Autodesk Inventor part; units mm, degrees
ref_plane "YZ Plane" through (0, 0, 0) normal (1, 0, 0) x (0, 1, 0)
ref_plane "XZ Plane" through (0, 0, 0) normal (0, 1, 0) x (-1, 0, 0)
ref_plane "XY Plane" through (0, 0, 0) normal (0, 0, 1) x (1, 0, 0)
sketch "Sketch1" plane through (0, 0, 0) normal (0, 1, 0) x (-1, 0, 0)
  line L0 (30, -20) -> (-30, -20)
  line L1 (-30, -20) -> (-30, 20)
  line L2 (-30, 20) -> (30, 20)
  line L3 (30, 20) -> (30, -20)
  line L4 (30, -20) -> (-30, 20) construction
  line L5 (-30, -20) -> (30, 20) construction
  point P0 (0, 0)
  dimension "d0" = 60
  dimension "d1" = 40
extrude "Extrusion1" add sketch "Sketch1" along normal blind 5.5
sketch "Sketch2" plane through (0, 5.5, 0) normal (0, 1, 0) x (1, 0, 0)
  line L0 (30, -20) -> (30, 20)
  line L1 (30, 0) -> (43.5, 0)
  line L2 (43.5, 0) -> (43.5, 10)
  line L3 (43.5, 10) -> (30, 10)
  line L4 (30, 10) -> (30, 0)
  line L5 (-43.1, 0) -> (48.6, 0)
  line L6 (43.5, 0) -> (43.5, -10)
  line L7 (43.5, -10) -> (30, -10)
  line L8 (30, -10) -> (30, 0)
  point P0 (0, 0)
  dimension "d4" = 13.5
  dimension "d5" = 10
extrude "Extrusion2" add sketch "Sketch2" against normal blind 5.5
sketch "Sketch3" plane through (0, 5.5, 0) normal (0, 1, 0) x (1, 0, 0)
  line L0 (43.5, 10) -> (30, 10)
  line L1 (30, 10) -> (30, 20)
  line L2 (35.5, 10) -> (38.5, 10)
  line L3 (38.5, 10) -> (38.5, 0)
  line L4 (38.5, 0) -> (35.5, 0)
  line L5 (35.5, 0) -> (35.5, 10)
  point P0 (0, 0)
  dimension "d8" = 5.5
  dimension "d9" = 3
  dimension "d10" = 10
extrude "Extrusion3" cut sketch "Sketch3" against normal through all
sketch "Sketch4" plane through (0, 5.5, 0) normal (0, 1, 0) x (1, 0, 0)
  line L0 (35.5, 0) -> (35.5, 10)
  line L1 (35.5, 10) -> (30, 10)
  line L2 (30, 10) -> (30, 20)
  line L3 (30, 20) -> (-30, 20)
  line L4 (-30, 20) -> (-30, -20)
  line L5 (-30, -20) -> (30, -20)
  line L6 (30, -20) -> (30, -10)
  line L7 (30, -10) -> (43.5, -10)
  line L8 (43.5, -10) -> (43.5, 10)
  line L9 (43.5, 10) -> (38.5, 10)
  line L10 (38.5, 10) -> (38.5, 0)
  line L11 (38.5, 0) -> (35.5, 0)
  point P0 (0, 0)
sketch "Sketch5" plane through (0, 5.5, 0) normal (0, 1, 0) x (1, 0, 0)
  line L0 (-30, 20) -> (-30, -20)
  line L1 (-44.7, 0) -> (58.2, 0)
  line L2 (0, 28) -> (0, -28)
  line L3 (-30, 0) -> (-41, 0)
  line L4 (-41, 0) -> (-41, 10)
  line L5 (-41, 10) -> (-30, 10)
  line L6 (-30, 10) -> (-30, 0)
  line L7 (-30, 0) -> (-41, 0)
  line L8 (-41, 0) -> (-41, -20)
  line L9 (-41, -20) -> (-30, -20)
  line L10 (-30, -20) -> (-30, 0)
  point P0 (0, 0)
  dimension "d14" = 11
  dimension "d15" = 10
extrude "Extrusion4" add sketch "Sketch5" against normal blind 5.5
sketch "Sketch6" plane through (0, 5.5, 0) normal (0, 1, 0) x (1, 0, 0)
  line L0 (-30, 20) -> (-30, 10)
  line L1 (-30, 10) -> (-41, 10)
  line L2 (-30, 0) -> (-35.5, 0)
  line L3 (-35.5, 0) -> (-35.5, 10)
  line L4 (-35.5, 10) -> (-30, 10)
  line L5 (-30, 10) -> (-30, 0)
  line L6 (-57.9, 0) -> (60.4, 0)
  line L7 (0, 28) -> (0, -28)
  point P0 (0, 0)
  dimension "d20" = 0
  dimension "d21" = 5.5
extrude "Extrusion5" cut sketch "Sketch6" against normal through all
equation "\"d2\" = Wt"
equation "\"d6\" = Wt"
equation "\"d8\" = Wt"
equation "\"d11\" = Wt"
equation "\"d14\" = 2 * Wt"
equation "\"d16\" = Wt"
equation "\"d21\" = Wt"
equation "\"d22\" = Wt"
properties part number "ex_holder_side" material "Wood (Birch)"
Source: CAD feature listing. Evaluate the final solid. Frame: model axes, mm. A direction names the side the tool comes from. Give positions to 0.01 mm unless a question says otherwise; leave off trailing zeros. Write each loop counter-clockwise with the first axis right and the second up, starting at its lowest first coordinate (ties: lowest second). Pieces come first, ordered by that corner, then holes. Notation, with made-up numbers: (71.25, 32) - (128.25, 32) arc R25 ccw to (128.25, 51) - close; hole circle Ø10 at (77, 58). An arc over 180 degrees is marked (long way). One line per item, written item: value. Start each with the question number.
Q1. Draft query along X for faces 4 (the face through (-33, 3, 0)), 5 (the face through (0, 3, -20)), 6 (the face through (30, 3, 15)), 7 (the face through (35.5, 3, -5)). Return one class per face: +X half, -X half, draft (parallel to the pull), parting line (faces both ways), or undercut.
Q2. Section query B-B, the plane x = 32. Return the cut outline in (y, z), then the cut area to 3 significant figures.
Q3. Section query A-A, the plane y = 2.85. Return the cut outline in (x, z), then the cut area to 4 significant figures.
Q4. Material intervals for probe 1 along X at (y, z) = (1.75, -0.5); probe 2 along X at (y, z) = (0.7, 11.5); probe 3 along Z at (x, y) = (-32, 3.8), sorted ascending. Write a range as from..to.
Q5. Set-up query: faces 1 (the face through (37, 3, 10)), 2 (the face through (-30, 3, -10)), 3 (the face through (30, 3, -15)). Return all of +Z, -Z, +X, -X, +Y, -Y with unobstructed straight access to the full face (end or side cutting, diameter ignored); none if empty.
Q6. First-contact query: pin 1 Ø3 at (y, z) = (2, -14.5) entering from -X; pin 2 Ø2 at (x, z) = (2.5, 5.5) entering from -Y; pin 3 Ø1.5 at (x, y) = (37, 3.5) entering from -Z; pin 4 Ø3 at (x, y) = (40, 2.5) entering from +Z. Flat tips, straight axial feed; report the tip coordinate or a pass-through.
Q7. Section query C-C, the plane z = -16. Return the cut outline in (x, y), then the cut area to 3 significant figures.
Answer:
1. face 4: undercut
1. face 5: draft
1. face 6: +X half
1. face 7: undercut
2. outline: (0, -10) - (5.5, -10) - (5.5, 10) - (0, 10) - close
2. area: 110 mm2
3. outline: (-41, -10) - (-35.5, -10) - (-35.5, 0) - (-30, 0) - (-30, -20) - (30, -20) - (30, -10) - (35.5, -10) - (35.5, 0) - (38.5, 0) - (38.5, -10) - (43.5, -10) - (43.5, 10) - (30, 10) - (30, 20) - (-41, 20) - close
3. area: 2,915 mm2
4. probe 1: x = -41..-35.5, -30..35.5, 38.5..43.5
4. probe 2: x = -41..30
4. probe 3: z = 0..20
5. face 1: +Z, +X, +Y, -Y
5. face 2: -Z, +Y, -Y
5. face 3: -Z, +X, +Y, -Y
6. pin 1: stops at x = -30
6. pin 2: stops at y = 0
6. pin 3: stops at z = 0
6. pin 4: stops at z = 10
7. outline: (-30, 0) - (30, 0) - (30, 5.5) - (-30, 5.5) - close
7. area: 330 mm2
